Design review of the part built by this model. Coordinates are the model's own, in mm. A direction names the side the tool comes from. Give positions to 0.01 mm unless a question says otherwise; leave off trailing zeros. Loops run counter-clockwise (first coordinate to the right, second up) from the corner with the lowest first, then second, coordinate; pieces in that order, holes last. Notation, with made-up numbers: (-33.75, 0) -> (-2.75, 0) arc R15 ccw to (-2.75, 22) -> close; hole circle Ø9 at (62, 71.25). An arc over 180 degrees is marked (long way). Use CSV: the item, a comma, the result in double quotes. Start each with the question number.
Item 1: We need section B-B (z = -67.5). State the section outline as (x, y) points (3 decimals), plus the area to 3 significant figures.
Item 2: We need section D-D (x = -77). State the section outline as (y, z) points (3 decimals).
Item 3: Wall thickness on line 1 along X through (y, z) = (37.5, -83); line 2 along Z through (x, y) = (127, 0); line 3 along X through (y, z) = (-49.5, 20): over which ranges is each line inside the solid? List them lowest first. Write a range as from..to.
Item 4: We need section A-A (y = 45). State the section outline as (x, z) points, plus the area to 3 significant figures.
Item 5: Clearance check with a flat-ended pin moving along its axis: pin 1 (2.5 mm diameter, centred on x = 15.5, y = -58, fed in from +Z). State where the tip first meets the part, or that it passes through.
Item 6: We need section C-C (y = 0). State the section outline as (x, z) points, plus the area to 3 significant figures.
Item 7: The part is to be moulded in two halves that separate along X. For faces 5 (the face through (129.517, -14.2, -24.3)), 6 (the face through (11, 53.98, -50)), 7 (the face through (-117.185, -1, -38)), say which applies: +X half, -X half, draft (parallel to the pull), parting line (faces both ways), or undercut.
Item 8: For faces 1 (the face through (123.146, -1, -46)), 2 (the face through (124, 0, 46.034)), 3 (the face through (12, -58, -8.219)), 4 (the face through (-109.748, -1, -38)), list the 3-axis set-ups (+Z, -Z, +X, -X, +Y, -Y) from which the entire face can be reached by the end or side of a thin tool; tool diameter is ignored.
from build123d import *

# Parameters (mm, degrees)
F1_DEPTH = 60
F4_W     = 68.7287449837
F4_H     = 109.1447398067
F5_DEPTH = 150.7
F2_W     = 232.8136488795
F2_H     = 109.1045513749
F6_DEPTH = 101.1
F7_W     = 58.0749809742
F7_H     = 110.2500036359
F8_DEPTH = 147.8
F9_D     = 30


with BuildPart() as f1:
    # F0 (on Front) → F1 (new body, symmetric)
    with BuildSketch(Plane.XZ):
        Polygon((-117.1853020787, 46.0337400436), (-117.1853020787, -92.6193669438), (129.5173019171, -92.6193669438), (129.5173019171, 46.0337400436), (64.2818138003, 46.0337400436), (64.2818138003, -8.2185808569), (-41.0197302699, -8.2185808569), (-41.0197302699, 46.0337400436), align=None)
    extrude(amount=F1_DEPTH, both=True)

    # F4 (on face) → F5 (cut)
    with BuildSketch(Plane.XY.offset(46.0337400436)):
        with Locations((-75.3841027617, -0.2763159573)):
            Rectangle(F4_W, F4_H)
    extrude(amount=-F5_DEPTH, mode=Mode.SUBTRACT)

    # F2 (on Top) → F6 (cut)
    with BuildSketch(Plane.XY):
        with Locations((6.7387260497, -0.5727261305)):
            Rectangle(F2_W, F2_H)
    extrude(amount=-F6_DEPTH, mode=Mode.SUBTRACT)

    # F7 (on face) → F8 (cut)
    with BuildSketch(Plane.XY.offset(46.0337400436)):
        with Locations((93.3193042874, 0)):
            Rectangle(F7_W, F7_H)
    extrude(amount=-F8_DEPTH, mode=Mode.SUBTRACT)

    # F9 (through all)
    with Locations(Plane.YZ.offset(129.5173019171)):
        with Locations((0, -18.2496998459)):
            Hole(F9_D / 2)


solid = f1.part
Results found:
1,outline,"(-117.185, -60) -> (129.517, -60) -> (129.517, 60) -> (-117.185, 60) -> close; hole (-109.748, -54.849) -> (-109.668, -54.849) -> (-109.668, -55.125) -> (123.146, -55.125) -> (123.146, 53.98) -> (122.357, 53.98) -> (122.357, 55.125) -> (64.282, 55.125) -> (64.282, 53.98) -> (-41.02, 53.98) -> (-41.02, 54.296) -> (-109.748, 54.296) -> close"
1,area,"4,110 mm²"
2,outline,"(-60, -92.619) -> (-55.125, -92.619) -> (-55.125, 0) -> (-54.849, 0) -> (-54.849, 46.034) -> (-60, 46.034) -> close; (54.296, -92.619) -> (60, -92.619) -> (60, 46.034) -> (54.296, 46.034) -> close"
3,line 1,"-117.19..-109.75, 123.15..129.52"
3,line 2,"-92.62..-33.25, -3.25..46.03"
3,line 3,"-117.19..-109.75, 122.36..129.52"
4,outline,"(-117.19, -92.62) -> (-109.75, -92.62) -> (-109.75, 46.03) -> (-117.19, 46.03) -> close; (122.36, 0) -> (123.15, 0) -> (123.15, -92.62) -> (129.52, -92.62) -> (129.52, 46.03) -> (122.36, 46.03) -> close"
4,area,"1,950 mm²"
5,pin 1,"z = -8.22"
6,outline,"(-117.19, -92.62) -> (-109.75, -92.62) -> (-109.75, -33.25) -> (-117.19, -33.25) -> close; (-117.19, -3.25) -> (-109.75, -3.25) -> (-109.75, 46.03) -> (-117.19, 46.03) -> close; (122.36, 0) -> (123.15, 0) -> (123.15, -3.25) -> (129.52, -3.25) -> (129.52, 46.03) -> (122.36, 46.03) -> close; (123.15, -92.62) -> (129.52, -92.62) -> (129.52, -33.25) -> (123.15, -33.25) -> close"
6,area,"1,540 mm²"
7,face 5,"+X half"
7,face 6,"undercut"
7,face 7,"-X half"
8,face 1,"-Z"
8,face 2,"+Z, +X, -X, +Y, -Y"
8,face 3,"+Z, +Y, -Y"
8,face 4,"+Z, -Z"
